from build123d import *

# Parameters (mm, degrees)
SKETCH1_W           = 20
SKETCH1_H           = 60
BOSS_EXTRUDE1_DEPTH = 5
SKETCH2_R           = 2.5
SKETCH2_R_2         = 1.25
BOSS_EXTRUDE2_DEPTH = 20
SKETCH3_R           = 1.25
CUT_EXTRUDE1_DEPTH  = 29
SKETCH4_R           = 2.5
SKETCH4_R_2         = 1.25
BOSS_EXTRUDE3_DEPTH = 20
SKETCH5_R           = 1.25
CUT_EXTRUDE2_DEPTH  = 29


with BuildPart() as part:
    # Sketch1 → Boss-Extrude1 (new body)
    with BuildSketch(Plane.XY):
        with Locations((10, 30)):
            Rectangle(SKETCH1_W, SKETCH1_H)
    extrude(amount=BOSS_EXTRUDE1_DEPTH)

    # Sketch2 → Boss-Extrude2 (add)
    with BuildSketch(Plane(origin=(20, 0, 0), x_dir=(0, 0, -1), z_dir=(1, 0, 0))):
        with Locations((-2.5, 60)):
            Circle(SKETCH2_R)
        with Locations((-2.5, 60)):
            Circle(SKETCH2_R_2, mode=Mode.SUBTRACT)
    extrude(amount=-BOSS_EXTRUDE2_DEPTH)

    # Sketch3 → Cut-Extrude1 (cut)
    with BuildSketch(Plane.ZY):
        with Locations((2.5, 60)):
            Circle(SKETCH3_R)
    extrude(amount=-CUT_EXTRUDE1_DEPTH, mode=Mode.SUBTRACT)

    # Sketch4 → Boss-Extrude3 (add)
    with BuildSketch(Plane.ZY):
        with Locations((2.5, 0)):
            Circle(SKETCH4_R)
        with Locations((2.5, 0)):
            Circle(SKETCH4_R_2, mode=Mode.SUBTRACT)
    extrude(amount=-BOSS_EXTRUDE3_DEPTH)

    # Sketch5 → Cut-Extrude2 (cut)
    with BuildSketch(Plane(origin=(20, 0, 0), x_dir=(0, 0, -1), z_dir=(1, 0, 0))):
        with Locations((-2.5, 0)):
            Circle(SKETCH5_R)
    extrude(amount=-CUT_EXTRUDE2_DEPTH, mode=Mode.SUBTRACT)


solid = part.part
Can you work these out from the model? Positions are in its coordinate system, mm. Give positions to 0.01 mm unless a question says otherwise; leave off trailing zeros. Loops run counter-clockwise (first coordinate to the right, second up) from the corner with the lowest first, then second, coordinate; pieces in that order, holes last. Notation, with made-up numbers: M 50,-10 L 104,-10 A14 ccw 104,2 Z; hole C -24,78 d3. An arc over 180 degrees is marked long. One line per item, written item: value. Start each with the question number.
1) I'm going to push flat-ended pins straight in: pin 1 (2 mm diameter, centred on y = 60, z = 2.5, fed in from +X); pin 2 (1.5 mm diameter, centred on x = 12, z = 1, fed in from -Y). Where does each tip first touch, or does it pass through?
2) If we section it at B-B, the plane x = 4.25: Write out the boundary of the cut face in (y, z), and give its area (3 significant figures).
3) Thinking about a two-plate mould opening in Z: for faces 1 (the face through (9.9, -2.5, 2.4)), 2 (the face through (9.86, -0.38, 1.31)), 3 (the face through (0, 30, 2)), 4 (the face through (9.86, 58.76, 2.66)), which applies, +Z half, -Z half, draft (parallel to the pull), parting line (faces both ways), or undercut?
4) If I drill on line 1 (Y direction, x = 13.5, z = 2.5); line 2 (Y direction, x = 17, z = 3.5); line 3 (Z direction, x = 13.25, y = 59.5), over which ranges is the centre line in solid material (lowest first)? Write a range as [from, to].
5) If we section it at A-A, the plane z = 2.5: Write out the boundary of the cut face in (x, y), and give its area (3 significant figures).
Completed:
1. pin 1: passes through
1. pin 2: stops at y = -2.38
2. outline: M 0,0 L 60,0 A2.5 ccw 60,5 L 0,5 A2.5 ccw Z; hole C 0,2.5 d2.5; hole C 60,2.5 d2.5
2. area: 310 mm^2
3. face 1: parting line
3. face 2: undercut
3. face 3: draft
3. face 4: undercut
4. line 1: y = [-2.5, -1.25], [1.25, 58.75], [61.25, 62.5]
4. line 2: y = [-2.29, -0.75], [0.75, 59.25], [60.75, 62.29]
4. line 3: z = [0, 1.35], [3.65, 5]
5. outline: M 0,-2.5 L 20,-2.5 L 20,-1.25 L 0,-1.25 Z; M 0,1.25 L 20,1.25 L 20,58.75 L 0,58.75 Z; M 0,61.25 L 20,61.25 L 20,62.5 L 0,62.5 Z
5. area: 1,200 mm^2
